The listing builds one solid part. Answer for the finished solid, in the listing's coordinates (mm). A direction names the side the tool comes from. Coordinates: 2 decimals unless noted, no trailing zeros. Order: outer loops, then holes, each group sorted by start corner. A loop starts at its lowest first (then second) coordinate and runs counter-clockwise, first axis right, second up. Notation, with made-up numbers: (73, -34) -> (112, -34) arc R3 ccw to (112, -29) -> close; hole circle Ø8 at (65.25, -38.75). An arc over 180 degrees is marked (long way). Answer in a Markdown table with one row per item. Add a question column.
```python
from build123d import *

# Parameters (mm, degrees)
BOSS_EXTRUDE1_DEPTH     = 2.5
CUT_EXTRUDE1_DEPTH      = 26.734218465
CUT_EXTRUDE2_DEPTH      = 26.734218465
BOSS_EXTRUDE2_DEPTH     = 2
BOSS_EXTRUDE3_DEPTH     = 2
CUT_EXTRUDE3_DEPTH      = 2
CUT_EXTRUDE3_DEPTH_BACK = 2
SKETCH9_W               = 3.535533906
SKETCH9_H               = 2
SKETCH9_H_2             = 4
CUT_EXTRUDE5_DEPTH      = 0.1
SKETCH10_W              = 20.9
SKETCH10_H              = 5.3
SKETCH10_H_2            = 5.296426242
SKETCH10_W_2            = 4.350252532
SKETCH10_H_3            = 16.8
CUT_EXTRUDE6_DEPTH      = 1.2
FILLET1_R               = 0.4


with BuildPart() as part:
    # Sketch1 → Boss-Extrude1 (new body)
    with BuildSketch(Plane.XY):
        Polygon((20, -1.5), (20, -8), (-20, -8), (-20, 8), (20, 8), (20, 1.5), (-5, 1.5), (-5, -1.5), align=None)
    extrude(amount=BOSS_EXTRUDE1_DEPTH)

    # Sketch2 → Cut-Extrude1 (cut, through all)
    with BuildSketch(Plane(origin=(0, 8, 0), x_dir=(1, 0, 0), z_dir=(0, 1, 0))):
        Polygon((20, -2.5), (17.5, 0), (20, 0), align=None)
    extrude(amount=-CUT_EXTRUDE1_DEPTH, mode=Mode.SUBTRACT)

    # Sketch5 → Cut-Extrude2 (cut, through all)
    with BuildSketch(Plane(origin=(0, 8, 0), x_dir=(1, 0, 0), z_dir=(0, 1, 0))):
        Polygon((-20, -2.5), (-17.5, 0), (-20, 0), align=None)
    extrude(amount=-CUT_EXTRUDE2_DEPTH, mode=Mode.SUBTRACT)

    # Sketch6 → Boss-Extrude2 (add)
    with BuildSketch(Plane(origin=(0, 8, 0), x_dir=(1, 0, 0), z_dir=(0, 1, 0))):
        Polygon((-12.550252532, 0), (-15.050252532, -2.5), (20, -2.5), (17.5, 0), align=None)
    extrude(amount=BOSS_EXTRUDE2_DEPTH)

    # Sketch7 → Boss-Extrude3 (add)
    with BuildSketch(Plane.XZ.offset(8)):
        Polygon((-12.550252532, 0), (17.5, 0), (20, 2.5), (-15.050252532, 2.5), align=None)
    extrude(amount=BOSS_EXTRUDE3_DEPTH)

    # Sketch8 → Cut-Extrude3 (cut, two sides: drawn at the far end of the back side and taken through both)
    with BuildSketch(Plane(origin=(0, 0, 0), x_dir=(1, 0, 0), z_dir=(0, 1, 0)).offset(-CUT_EXTRUDE3_DEPTH_BACK)):
        Polygon((-15.050252532, -2.5), (-12.550252532, 0), (-17.5, 0), (-20, -2.5), align=None)
    extrude(amount=CUT_EXTRUDE3_DEPTH + CUT_EXTRUDE3_DEPTH_BACK, mode=Mode.SUBTRACT)

    # Sketch9 → Cut-Extrude5 (cut)
    with BuildSketch(Plane(origin=(-6.275126266, 0, -6.275126266), x_dir=(-0.7071067811865476, 0, 0.7071067811865476), z_dir=(-0.7071067811865476, 0, -0.7071067811865476))):
        with Locations((10.642135624, 9)):
            Rectangle(SKETCH9_W, SKETCH9_H)
        with Locations((10.642135624, 0)):
            Rectangle(SKETCH9_W, SKETCH9_H_2)
        with Locations((10.642135624, -9)):
            Rectangle(SKETCH9_W, SKETCH9_H)
    extrude(amount=-CUT_EXTRUDE5_DEPTH, mode=Mode.SUBTRACT)

    # Sketch10 → Cut-Extrude6 (cut)
    with BuildSketch(Plane(origin=(0, 0, 0), x_dir=(-1, 0, 0), z_dir=(0, 0, -1))):
        with Locations((-5.45, -5.75)):
            Rectangle(SKETCH10_W, SKETCH10_H)
        with Locations((-5.45, 5.751786879)):
            Rectangle(SKETCH10_W, SKETCH10_H_2)
        with Locations((8.775126266, 0)):
            Rectangle(SKETCH10_W_2, SKETCH10_H_3)
    extrude(amount=-CUT_EXTRUDE6_DEPTH, mode=Mode.SUBTRACT)

    # Fillet1
    fillet1_edges = [part.edges().sort_by_distance(p)[0] for p in [
        (-5, 1.5, 1.25),
        (-5, -1.5, 1.25),
        (-10.950252532, 8.4, 0.6),
        (-10.950252532, -8.4, 0.6),
        (-6.6, -8.4, 0.6),
        (-6.6, 8.4, 0.6),
        (-5, 8.4, 0.6),
        (-5, 3.103573758, 0.6),
        (15.9, 3.103573758, 0.6),
        (15.9, 8.4, 0.6),
        (15.9, -8.4, 0.6),
        (15.9, -3.1, 0.6),
        (-5, -3.1, 0.6),
        (-5, -8.4, 0.6),
        (18.75, -1.5, 1.25),
        (18.75, 1.5, 1.25),
        (18.75, 10, 1.25),
        (18.75, -10, 1.25),
    ]]
    fillet(fillet1_edges, radius=FILLET1_R)


solid = part.part
```
Q1. Given pin 1 (1.3 mm diameter, centred on x = -18, z = 0.5, fed in from +Y); pin 2 (2.5 mm diameter, centred on x = 8.5, y = -6.5, fed in from -Z); pin 3 (1.2 mm diameter, centred on x = -17.5, z = 1.5, fed in from -Y); pin 4 (3 mm diameter, centred on x = 4.5, y = -4, fed in from -Z), each flat-ended and moving along its own axis, determine where each tip first touches the part or whether it passes through.
Q2. A cutting plane is placed at B-B (y = -0.25). Determine the outline of the cut face in (x, z), then the cut area to 3 significant figures.
Q3. A cutting plane is placed at D-D (x = -13.5). Determine the outline of the cut face in (y, z), then the cut area to 3 significant figures.
Q4. A cutting plane is placed at A-A (x = -4). Determine the outline of the cut face in (y, z), then the cut area to 3 significant figures.
Q5. A cutting plane is placed at C-C (y = -6). Determine the outline of the cut face in (x, z), then the cut area to 3 significant figures.
Q6. For faces 4 (the face through (8, 1.5, 1)), 5 (the face through (-5, -6, 1)), 6 (the face through (18.543, 1.614, 1.213)), determine the directions among +Z, -Z, +X, -X, +Y, -Y from which every point of the face is accessible in a straight line to the end or side of a thin tool.
Q7. Determine the mould class of faces 1 (the face through (18.51, 9.88, 1.17)), 2 (the face through (6, -8.4, 1)), 3 (the face through (-18.8, 5, 1.3)) for opening direction Y: +Y half, -Y half, draft (parallel to the pull), parting line (faces both ways), or undercut.
Q8. Straight lines are drawn through the part: line 1 (Y direction, x = 2, z = 0.2); line 2 (Y direction, x = -17, z = 0.8); line 3 (X direction, y = 6.75, z = 0.75). For each, find the intervals that lie inside material, in ascending order.
Returned:
| question | item | result |
|---|---|---|
| 1 | pin 1 | stops at y = 8 |
| 1 | pin 2 | stops at z = 1.2 |
| 1 | pin 3 | stops at y = -8 |
| 1 | pin 4 | stops at z = 0 |
| 2 | outline | (-14.91, 2.5) -> (-12.48, 0.07) -> (-12.55, 0) -> (-10.95, 0) -> (-10.95, 1.2) -> (-6.6, 1.2) -> (-6.6, 0) -> (-5, 0) -> (-5, 2.5) -> close |
| 2 | area | 16.4 mm² |
| 3 | outline | (-10, 1.09) -> (-8, 1.09) -> (-8, 0) -> (-2, 0) -> (-2, 1.09) -> (2, 1.09) -> (2, 0) -> (8, 0) -> (8, 1.09) -> (10, 1.09) -> (10, 2.5) -> (-10, 2.5) -> close |
| 3 | area | 41.3 mm² |
| 4 | outline | (-10, 0) -> (-8.4, 0) -> (-8.4, 1.2) -> (-3.1, 1.2) -> (-3.1, 0) -> (-1.5, 0) -> (-1.5, 2.5) -> (-10, 2.5) -> close; (1.5, 0) -> (3.1, 0) -> (3.1, 1.2) -> (8.4, 1.2) -> (8.4, 0) -> (10, 0) -> (10, 2.5) -> (1.5, 2.5) -> close |
| 4 | area | 29.8 mm² |
| 5 | outline | (-20, 2.5) -> (-17.5, 0) -> (-10.95, 0) -> (-10.95, 1.2) -> (-6.6, 1.2) -> (-6.6, 0) -> (-5, 0) -> (-5, 1.2) -> (15.9, 1.2) -> (15.9, 0) -> (17.5, 0) -> (20, 2.5) -> close |
| 5 | area | 63.4 mm² |
| 6 | face 4 | +Z, -Z, +X |
| 6 | face 5 | -Z |
| 6 | face 6 | -Z, +X |
| 7 | face 1 | +Y half |
| 7 | face 2 | undercut |
| 7 | face 3 | draft |
| 8 | line 1 | y = -10 to -8.4, -3.1 to -1.5, 1.5 to 3.1, 8.4 to 10 |
| 8 | line 2 | y = -8 to -2, 2 to 8 |
| 8 | line 3 | x = -18.25 to -10.95, -6.6 to -5, 15.9 to 18.25 |
